from build123d import *

# Parameters (mm, degrees)
BASPROSKE_W             = 5
BASPROSKE_H             = 5.5
TOOTHCUT_DEPTH          = 10.246621004
TEETHCUTS_COUNT         = 20
TEETHCUTS_ANGLE         = 342
BORSKE_R                = 0.5
BORE_DEPTH              = 50.0000508
CUT_EXTRUDE1_DEPTH      = 10.188413972
CUT_EXTRUDE1_DEPTH_BACK = 10.188413972


with BuildPart() as part:
    # BasProSke → Base-Revolve (revolve)
    with BuildSketch(Plane(origin=(0, 0, 0), x_dir=(1, 0, 0), z_dir=(0, 1, 0)), mode=Mode.PRIVATE) as base_revolve_sk:
        with Locations((2.5, 2.75)):
            Rectangle(BASPROSKE_W, BASPROSKE_H)
    revolve(base_revolve_sk.sketch.rotate(Axis((-10, 0, 0), (1, 0, 0)), 180), axis=Axis((-10, 0, 0), (1, 0, 0)))

    # TooCutSke → ToothCut (cut, through all)
    with BuildSketch(Plane(origin=(0, 0, 0), x_dir=(0, 0, -1), z_dir=(1, 0, 0))):
        with BuildLine():
            ThreePointArc((0.249903181, 4.366855207), (0, 4.374), (-0.249903181, 4.366855207))
            ThreePointArc((-0.249903181, 4.366855207), (-0.415207844, 4.95951031), (-0.752843848, 5.473871692))
            ThreePointArc((-0.752843848, 5.473871692), (0, 5.5254), (0.752843848, 5.473871692))
            ThreePointArc((0.752843848, 5.473871692), (0.415207844, 4.95951031), (0.249903181, 4.366855207))
        make_face()
    toothcut = extrude(amount=TOOTHCUT_DEPTH, mode=Mode.SUBTRACT)

    # TeethCuts: ToothCut ×20 about axis
    teethcuts_axis = Axis((-10, 0, 0), (1, 0, 0))
    for i in range(1, TEETHCUTS_COUNT):
        add(toothcut.rotate(teethcuts_axis, i * TEETHCUTS_ANGLE / (TEETHCUTS_COUNT - 1)), mode=Mode.SUBTRACT)

    # BorSke → Bore (cut, symmetric)
    with BuildSketch(Plane(origin=(0, 0, 0), x_dir=(0, 0, -1), z_dir=(1, 0, 0))):
        with Locations(Location((0, 0, 0), (0, 0, 180))):
            Circle(BORSKE_R)
    extrude(amount=BORE_DEPTH, both=True, mode=Mode.SUBTRACT)

    # Sketch1 → Cut-Extrude1 (cut, two sides)
    with BuildSketch(Plane(origin=(5, 0, 0), x_dir=(0, 0, -1), z_dir=(1, 0, 0))) as cut_extrude1_sk:
        with BuildLine():
            Line((1.25, -1.759357098), (-1.25, -1.759357098))
            Line((-1.25, -1.759357098), (-1.25, -2.449489743))
            ThreePointArc((-1.25, -2.449489743), (0, -2.75), (1.25, -2.449489743))
            Line((1.25, -2.449489743), (1.25, -1.759357098))
        make_face()
        with BuildLine():
            Line((-1.25, -2.449489743), (-1.25, -1.759357098))
            Line((-1.25, -1.759357098), (1.25, -1.759357098))
            Line((1.25, -1.759357098), (1.25, -2.449489743))
            ThreePointArc((1.25, -2.449489743), (2.34520788, -1.436140662), (2.75, 0))
            ThreePointArc((2.75, 0), (-1.436140662, 2.34520788), (-1.25, -2.449489743))
        make_face()
        with BuildLine():
            ThreePointArc((1.25, -2.449489743), (0, -2.75), (-1.25, -2.449489743))
            Line((-1.25, -2.449489743), (-1.25, -3.5))
            Line((-1.25, -3.5), (1.25, -3.5))
            Line((1.25, -3.5), (1.25, -2.449489743))
        make_face()
    extrude(amount=CUT_EXTRUDE1_DEPTH, mode=Mode.SUBTRACT)
    extrude(cut_extrude1_sk.sketch, amount=-CUT_EXTRUDE1_DEPTH_BACK, mode=Mode.SUBTRACT)


solid = part.part
Design review of the part built by this model. Coordinates are the model's own, in mm. A direction names the side the tool comes from. Coordinates: 2 decimals unless noted, no trailing zeros. Write each loop counter-clockwise with the first axis right and the second up, starting at its lowest first coordinate (ties: lowest second). Pieces come first, ordered by that corner, then holes. Notation, with made-up numbers: (46.5, 36.25) -> (54.5, 36.25) arc R18 cw to (54.5, 68.25) -> close; hole circle Ø1 at (37.5, -17.75). An arc over 180 degrees is marked (long way). Write each question's results on one line, items separated by ' | '. Start each with the question number.
(1) Take a section at B-B on y = -2. Write out the cut boundary in (x, z).
(2) Clearance check with flat-ended pins moving along their axes: P1, Ø1.5, axis at x = 2, y = -2, coming from the -Z side; P2, Ø6.5, axis at y = 0, z = 0, coming from the -X side; P3, Ø0.5, axis at x = 1.5, y = -3, coming from the -Z side. State where each tip first meets the part, or that it passes through.
(3) For line 1 along Y through (x, z) = (0.8, -0.75); line 2 along Y through (x, z) = (2, 1.75); line 3 along Z through (x, y) = (1.75, -2), list the stretches that pass through material, from the lowest coordinate up. Write a range as from..to.
(4) Take a section at A-A on z = 0. Write out the cut boundary in (x, y), and give its area (3 significant figures).
(5) Tool access review of faces 5 (the face through (2.465, 0.406, -4.938)), 6 (the face through (2.46, -4.57, -1.91)), 7 (the face through (2.46, -1.14, -4.82)), 8 (the face through (2.465, 3.765, -3.245)): name each direction out of +Z, -Z, +X, -X, +Y, -Y from which nothing blocks a thin tool from reaching the whole face with its end or side.
(6) The part is to be moulded in two halves that separate along Y. For faces 1 (the face through (5, 2.3, -2.3)), 2 (the face through (2.465, 2.574, 4.233)), 3 (the face through (2.46, 4.57, 1.91)), 4 (the face through (2.465, -3.756, -3.23)), say which applies: pulls with the +Y half, pulls with the -Y half, needs draft (parallel to the pull), parting line crosses it, or undercut.
Results found:
1) outline: (0, -4.66) -> (5, -4.66) -> (5, -1.89) -> (0, -1.89) -> close; (0, 1.89) -> (5, 1.89) -> (5, 4.66) -> (0, 4.66) -> close
2) P1: stops at z = -4.96 | P2: stops at x = 0 | P3: stops at z = -3.77
3) line 1: y = -5.45..-3.5, 2.65..5.45 | line 2: y = -4.36..-2.12, 2.12..4.36 | line 3: z = -4.66..-1.89, 1.89..4.66
4) outline: (0, -4.37) -> (5, -4.37) -> (5, -3.5) -> (0, -3.5) -> close; (0, 2.75) -> (5, 2.75) -> (5, 4.37) -> (0, 4.37) -> close | area: 12.5 mm2
5) face 5: -Z, +X, -X | face 6: +X, -X, -Y | face 7: +X, -X | face 8: +X, -X, +Y
6) face 1: needs draft | face 2: undercut | face 3: pulls with the +Y half | face 4: pulls with the -Y half
